Study the drawing (mm; zero at the part's minimum x, y, z) and answer. Coordinates: 2 decimals unless noted, no trailing zeros. Loops run counter-clockwise (first coordinate to the right, second up) from the corner with the lowest first, then second, coordinate; pieces in that order, holes last. Notation, with made-up numbers: (29.5, -23) - (44.5, -23) arc R27 ccw to (44.5, -6) - close; hole circle Ø3 at (-3.5, -8.75). An arc over 180 degrees is marked (long way). Put each result on its own line as item: value.
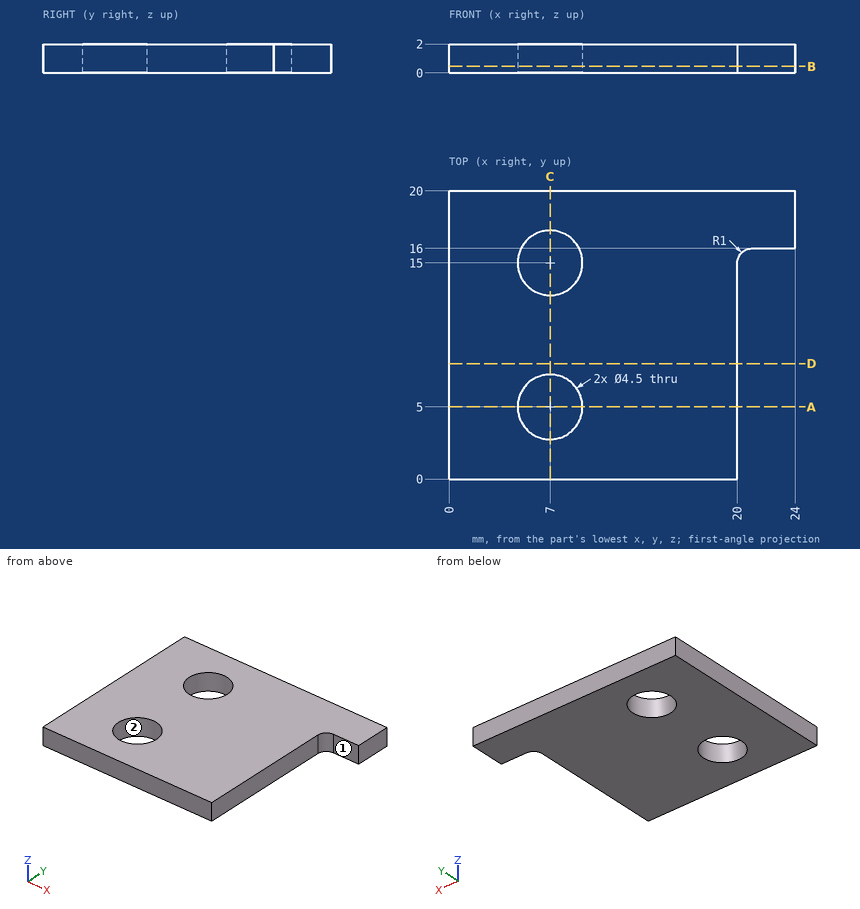
1) For a pull along X with two mould halves and no side action, classify the marked faces 1 and 2 as pulls with the +X half, pulls with the -X half, needs draft (parallel to the pull), parting line crosses it, or undercut.
Found:
face 1: needs draft
face 2: undercut
2) The part is cut by section A-A (y = 5). Give the vertices of the cut face in (x, z).
Found:
outline: (0, 0) - (4.75, 0) - (4.75, 2) - (0, 2) - close; (9.25, 0) - (20, 0) - (20, 2) - (9.25, 2) - close
3) The part is cut by section B-B (z = 0.45). Give the vertices of the cut face in (x, y), and give its area (3 significant figures).
Found:
outline: (0, 0) - (20, 0) - (20, 15) arc R1 cw to (21, 16) - (24, 16) - (24, 20) - (0, 20) - close; hole circle Ø4.5 at (7, 5); hole circle Ø4.5 at (7, 15)
area: 384 mm^2
4) The part is cut by section D-D (y = 8). Give the vertices of the cut face in (x, z), and give its area (3 significant figures).
Found:
outline: (0, 0) - (20, 0) - (20, 2) - (0, 2) - close
area: 40.0 mm^2
5) The part is cut by section C-C (x = 7). Give the vertices of the cut face in (y, z).
Found:
outline: (0, 0) - (2.75, 0) - (2.75, 2) - (0, 2) - close; (7.25, 0) - (12.75, 0) - (12.75, 2) - (7.25, 2) - close; (17.25, 0) - (20, 0) - (20, 2) - (17.25, 2) - close
6) Straight lines are drawn through the part: L1, parallel to Y at x = 7, z = 0.5; L2, parallel to X at y = 5, z = 1.3; L3, parallel to Y at x = 6, z = 1.35. For each, find the intervals that lie inside material, in ascending order. Write a range as [from, to].
Found:
L1: y = [0, 2.75], [7.25, 12.75], [17.25, 20]
L2: x = [0, 4.75], [9.25, 20]
L3: y = [0, 2.98], [7.02, 12.98], [17.02, 20]
